from build123d import *

# Parameters (mm, degrees)
F0_R     = 1.25
F0_R_2   = 1.55
F1_DEPTH = 4
F6_W     = 32
F6_H     = 52
F7_DEPTH = 2
F8_W     = 28
F8_H     = 48.26
F9_DEPTH = 4


with BuildPart() as f1:
    # F0 (on Top) → F1 (new body)
    with BuildSketch(Plane.XY):
        Polygon((-13.626695, 74.19249), (-31.626695, 74.19249), (-61.326636, 24.569767), (-61.326636, -0.930233), (-70.126636, -0.930233), (-70.126636, -15.930233), (-61.326636, -15.930233), (-61.326636, -20.930233), (16.073364, -20.930233), (16.073364, -15.930233), (24.873364, -15.930233), (24.873364, -0.930233), (16.073246, -0.930233), (16.073246, 24.569767), align=None)
        with Locations((-57.026636, -16.630233)):
            Circle(F0_R, mode=Mode.SUBTRACT)
        with Locations((-57.026636, 1.369767)):
            Circle(F0_R, mode=Mode.SUBTRACT)
        with Locations((-48.186636, 3.339767)):
            Circle(F0_R_2, mode=Mode.SUBTRACT)
        with Locations((0.073364, 2.069767)):
            Circle(F0_R_2, mode=Mode.SUBTRACT)
        with Locations((11.773364, -16.630233)):
            Circle(F0_R, mode=Mode.SUBTRACT)
        with Locations((11.116156, 1.369767)):
            Circle(F0_R, mode=Mode.SUBTRACT)
        with Locations((-32.946636, 54.139767)):
            Circle(F0_R_2, mode=Mode.SUBTRACT)
        with Locations((-29.159842, 66.82249)):
            Circle(F0_R, mode=Mode.SUBTRACT)
        with Locations((-5.006636, 54.139767)):
            Circle(F0_R_2, mode=Mode.SUBTRACT)
        with Locations((-14.419842, 66.82249)):
            Circle(F0_R, mode=Mode.SUBTRACT)
    extrude(amount=F1_DEPTH)

    # F6 (on face) → F7 (join)
    with BuildSketch(Plane.XY.offset(4)):
        with Locations((-22.18772, 5.069767)):
            Rectangle(F6_W, F6_H)
    extrude(amount=F7_DEPTH)

    # F8 (on face) → F9 (cut)
    with BuildSketch(Plane.XY.offset(6)):
        with Locations((-22.18772, 5.199767)):
            Rectangle(F8_W, F8_H)
    extrude(amount=-F9_DEPTH, mode=Mode.SUBTRACT)


with BuildPart() as f2_1:
    # F2: copy of F1
    add(f1.part.moved(Location((0, 0, 7))))


with BuildPart() as f4_1:
    # F4: copy of F1
    add(f1.part.moved(Location((0, 0, 6))))


solid = f1.part
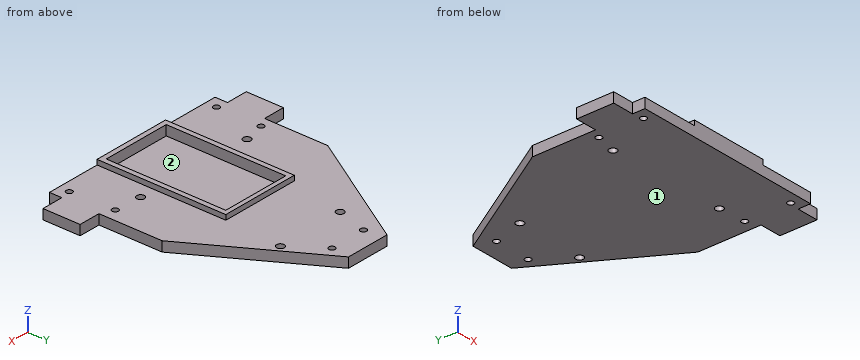
Could you check a few things on this model? Use its own coordinates, in mm. Face numbers are marked on the shaded views. Give positions to 0.01 mm unless a question says otherwise; leave off trailing zeros. Write each loop counter-clockwise with the first axis right and the second up, starting at its lowest first coordinate (ties: lowest second). Pieces come first, ordered by that corner, then holes. Notation, with made-up numbers: (31.25, 87) -> (38.25, 87) arc R22 ccw to (38.25, 113) -> close; hole circle Ø6 at (2, -32.5). An arc over 180 degrees is marked (long way). Answer as a JSON object with one key per item and string values.
Q1. Suppose I cut it at B-B on x = -21.5. Write out the boundary of the cut face in (y, z).
Taken from the geometry:
{"outline": "(-20.93, 0) -> (74.19, 0) -> (74.19, 4) -> (31.07, 4) -> (31.07, 6) -> (29.33, 6) -> (29.33, 2) -> (-18.93, 2) -> (-18.93, 6) -> (-20.93, 6) -> close"}
Q2. We'd pull the mould along X, two halves only. Please class the marked faces 1 and 2: released by +X, released by -X, zero draft, split by the parting line, or undercut.
Taken from the geometry:
{"face 1": "zero draft", "face 2": "undercut"}
Q3. Suppose I cut it at A-A on y = -12.5. Write out the boundary of the cut face in (x, z).
Taken from the geometry:
{"outline": "(-70.13, 0) -> (24.87, 0) -> (24.87, 4) -> (-6.19, 4) -> (-6.19, 6) -> (-8.19, 6) -> (-8.19, 2) -> (-36.19, 2) -> (-36.19, 6) -> (-38.19, 6) -> (-38.19, 4) -> (-70.13, 4) -> close"}
Q4. Suppose I cut it at C-C on z = 1.05. Count the separate pieces of the cut face and the enclosed holes in it, then the cut area to 3 significant figures.
Taken from the geometry:
{"separate pieces": "1", "enclosed holes": "10", "area": "6,090 mm²"}
Q5. Suppose I cut it at D-D on y = 14. Write out the boundary of the cut face in (x, z), then the cut area to 3 significant figures.
Taken from the geometry:
{"outline": "(-61.33, 0) -> (16.07, 0) -> (16.07, 4) -> (-6.19, 4) -> (-6.19, 6) -> (-8.19, 6) -> (-8.19, 2) -> (-36.19, 2) -> (-36.19, 6) -> (-38.19, 6) -> (-38.19, 4) -> (-61.33, 4) -> close", "area": "262 mm²"}
Q6. Please list where these lines run through material, in increasing order: L1, parallel to Y at x = -31, z = 5.7; L2, parallel to X at y = 2, z = 5.15; L3, parallel to Y at x = -24, z = 3.1.
Taken from the geometry:
{"L1": "y = -20.93 to -18.93, 29.33 to 31.07", "L2": "x = -38.19 to -36.19, -8.19 to -6.19", "L3": "y = -20.93 to -18.93, 29.33 to 74.19"}
Q7. Will these pins go through, and if not, where does the flat tip stop? pin 1 Ø6 at (x, y) = (-3, 8) entering from -Z; pin 2 Ø3 at (y, z) = (58.5, 4.5) entering from +X; pin 3 Ø3 at (x, y) = (-57.03, -16.63) entering from +Z; pin 4 Ø14 at (x, y) = (-19, 14.5) entering from +Z.
Taken from the geometry:
{"pin 1": "stops at z = 0", "pin 2": "stops at x = -3.39", "pin 3": "stops at z = 4", "pin 4": "stops at z = 2"}
